```python
from build123d import *

# Parameters (mm, degrees)
SKETCH1_W                   = 89
SKETCH1_H                   = 83
SKETCH1_R                   = 1.3
MAIN_BODY_DEPTH             = 14
SKETCH2_W                   = 73.025
SKETCH2_H                   = 83
SKETCH2_R                   = 4
SCREW_RISER_DEPTH           = 2
SKETCH4_W                   = 7.9875
SKETCH4_H                   = 83
TOPPER_SUPPORT_DEPTH        = 20
MOUNT_START                 = -44.5
MOUNT_NUTS_DEPTH            = 41.275
F_9_32_MOUNT_HOLES_REACH    = 9.988
SKETCH5_R                   = 3.3734375
SKETCH8_W                   = 19.0125
SKETCH8_H                   = 43
MIDDLE_CUT_DEPTH            = 14
SKETCH9_R                   = 3.3734375
MOUNT_NUTS_P2_DEPTH         = 4.7625
SKETCH9_3_R                 = 3.3734375
F_9_32_MOUNT_HOLES_P2_DEPTH = 7.9875


with BuildPart() as part:
    # Sketch1 → Main Body (new body)
    with BuildSketch(Plane(origin=(0, 0, 0), x_dir=(1, 0, 0), z_dir=(0, 1, 0))):
        with Locations((0, 41.5)):
            Rectangle(SKETCH1_W, SKETCH1_H)
        with Locations((-30, 14.25)):
            Circle(SKETCH1_R, mode=Mode.SUBTRACT)
        with Locations((30, 14.25)):
            Circle(SKETCH1_R, mode=Mode.SUBTRACT)
        with BuildLine():
            Line((-7.5, 12.5), (-7.5, 70.5))
            ThreePointArc((-7.5, 70.5), (0, 78), (7.5, 70.5))
            Line((7.5, 70.5), (7.5, 12.5))
            ThreePointArc((7.5, 12.5), (0, 5), (-7.5, 12.5))
        make_face(mode=Mode.SUBTRACT)
        with Locations((-30, 68.75)):
            Circle(SKETCH1_R, mode=Mode.SUBTRACT)
        with Locations((30, 68.75)):
            Circle(SKETCH1_R, mode=Mode.SUBTRACT)
    extrude(amount=MAIN_BODY_DEPTH)

    # Sketch2 → Screw Riser (cut)
    with BuildSketch(Plane(origin=(0, 14, 0), x_dir=(1, 0, 0), z_dir=(0, 1, 0))):
        with Locations((0, 41.5)):
            Rectangle(SKETCH2_W, SKETCH2_H)
        with Locations((-30, 14.25)):
            Circle(SKETCH2_R, mode=Mode.SUBTRACT)
        with Locations((30, 14.25)):
            Circle(SKETCH2_R, mode=Mode.SUBTRACT)
        with Locations((-30, 68.75)):
            Circle(SKETCH2_R, mode=Mode.SUBTRACT)
        with Locations((30, 68.75)):
            Circle(SKETCH2_R, mode=Mode.SUBTRACT)
    extrude(amount=-SCREW_RISER_DEPTH, mode=Mode.SUBTRACT)

    # Sketch4 → Topper Support (add)
    with BuildSketch(Plane(origin=(0, 14, 0), x_dir=(1, 0, 0), z_dir=(0, 1, 0))):
        with Locations((-40.50625, 41.5)):
            Rectangle(SKETCH4_W, SKETCH4_H)
        with Locations((40.50625, 41.5)):
            Rectangle(SKETCH4_W, SKETCH4_H)
    extrude(amount=TOPPER_SUPPORT_DEPTH)

    # Sketch6 → Mount Nuts (cut)
    with BuildSketch(Plane.ZY.offset(44.5).offset(MOUNT_START)):
        Polygon((-52.96962719, 22.65546875), (-56.234813595, 28.3109375), (-62.765186405, 28.3109375), (-66.03037281, 22.65546875), (-62.765186405, 17), (-56.234813595, 17), align=None)
        Polygon((-16.96962719, 22.65546875), (-20.234813595, 28.3109375), (-26.765186405, 28.3109375), (-30.03037281, 22.65546875), (-26.765186405, 17), (-20.234813595, 17), align=None)
    extrude(amount=MOUNT_NUTS_DEPTH, mode=Mode.SUBTRACT)

    # Sketch5 → 9/32 Mount Holes (cut, up to next)
    with BuildSketch(Plane.ZY.offset(36.5125), mode=Mode.PRIVATE) as f_9_32_mount_holes_sk1:
        with Locations((-59.5, 22.65546875)):
            Circle(SKETCH5_R)
    f_9_32_mount_holes_tool1 = extrude(f_9_32_mount_holes_sk1.sketch, amount=F_9_32_MOUNT_HOLES_REACH, mode=Mode.PRIVATE) & part.part
    add(f_9_32_mount_holes_tool1.solids().sort_by_distance((-36.5125, 22.655469, -59.5))[0], mode=Mode.SUBTRACT)
    # Sketch5 → 9/32 Mount Holes (cut, up to next)
    with BuildSketch(Plane.ZY.offset(36.5125), mode=Mode.PRIVATE) as f_9_32_mount_holes_sk2:
        with Locations((-23.5, 22.65546875)):
            Circle(SKETCH5_R)
    f_9_32_mount_holes_tool2 = extrude(f_9_32_mount_holes_sk2.sketch, amount=F_9_32_MOUNT_HOLES_REACH, mode=Mode.PRIVATE) & part.part
    add(f_9_32_mount_holes_tool2.solids().sort_by_distance((-36.5125, 22.655469, -23.5))[0], mode=Mode.SUBTRACT)

    # Sketch8 → Middle Cut (cut)
    with BuildSketch(Plane(origin=(0, 14, 0), x_dir=(1, 0, 0), z_dir=(0, 1, 0))):
        with Locations((-27.00625, 41.5)):
            Rectangle(SKETCH8_W, SKETCH8_H)
        with Locations((27.00625, 41.5)):
            Rectangle(SKETCH8_W, SKETCH8_H)
    extrude(amount=-MIDDLE_CUT_DEPTH, mode=Mode.SUBTRACT)

    # Sketch9 → Mount Nuts p2 (cut)
    with BuildSketch(Plane.ZY.offset(-36.5125)):
        Polygon((-56.234813595, 17), (-62.765186405, 17), (-66.03037281, 22.65546875), (-62.765186405, 28.3109375), (-56.234813595, 28.3109375), (-52.96962719, 22.65546875), align=None)
        with Locations((-59.5, 22.65546875)):
            Circle(SKETCH9_R, mode=Mode.SUBTRACT)
        with Locations((-59.5, 22.65546875)):
            Circle(SKETCH9_R)
        Polygon((-20.234813595, 17), (-26.765186405, 17), (-30.03037281, 22.65546875), (-26.765186405, 28.3109375), (-20.234813595, 28.3109375), (-16.96962719, 22.65546875), align=None)
        with Locations((-23.5, 22.65546875)):
            Circle(SKETCH9_R, mode=Mode.SUBTRACT)
        with Locations((-23.5, 22.65546875)):
            Circle(SKETCH9_R)
    extrude(amount=-MOUNT_NUTS_P2_DEPTH, mode=Mode.SUBTRACT)

    # Sketch9<3> → 9/32 Mount Holes p2 (cut)
    with BuildSketch(Plane.ZY.offset(-36.5125)):
        with Locations((-59.5, 22.65546875)):
            Circle(SKETCH9_3_R)
        with Locations((-23.5, 22.65546875)):
            Circle(SKETCH9_3_R)
    extrude(amount=-F_9_32_MOUNT_HOLES_P2_DEPTH, mode=Mode.SUBTRACT)


solid = part.part
```
Model file for the job. Use its own axes, mm. A direction names the side the tool comes from. Coordinates: 2 decimals unless noted, no trailing zeros. Write each loop counter-clockwise with the first axis right and the second up, starting at its lowest first coordinate (ties: lowest second). Pieces come first, ordered by that corner, then holes. Notation, with made-up numbers: (-3, 49) - (1, 49) arc R12 ccw to (1, 55) - close; hole circle Ø4 at (79.5, 55.25). An arc over 180 degrees is marked (long way). One line per item, written item: value. Start each with the question number.
1. Mould opens along X. For faces 4 (the flat face through (36.512, 17, -41)), 5 (the flat face through (44.5, 17, -41)), 6 (the flat face through (17.5, 6, -41)), 7 (the flat face through (40, 34, -42)) say: released by +X, released by -X, zero draft, split by the parting line, or undercut.
2. Tool access for faces 1 (the flat face through (-27, 6, -63)), 2 (the flat face through (-41.275, 20, -57)), 3 (the cylindrical face through (42.865, 21.363, -56.384)): list every direction of +Z, -Z, +X, -X, +Y, -Y with a clear straight run to the whole face (end or side of a thin tool).
3. Flat gauge pins, fed straight in: pin 1 (5.5 mm diameter, centred on y = 22.66, z = -59.5, fed in from -X); pin 2 (10 mm diameter, centred on x = 8.5, z = -21.5, fed in from +Y); pin 3 (9 mm diameter, centred on x = 29, z = -13, fed in from +Y). Where does each tip first touch, or does it go through?
4. Slice it at A-A (x = 30). Write the cut outline in (y, z), plus the area to 3 significant figures.
5. Slice it at B-B (z = -23.5). Count the separate pieces of the cut face and the enclosed holes in it, plus the area to 3 significant figures.
6. Probe line 1 (X direction, y = 9.5, z = -14.25); line 2 (X direction, y = 3.5, z = -22); line 3 (Z direction, x = -30, y = 4). List the from-to ranges inside material, lowest first. Write a range as from..to.
7. Slice it at C-C (x = 0). Write the cut outline in (y, z).
8. Slice it at D-D (y = 3). Write the cut outline in (x, z).
Answers below:
1. face 4: undercut
1. face 5: released by +X
1. face 6: undercut
1. face 7: zero draft
2. face 1: +Y, -Y
2. face 2: none
2. face 3: +X, -X
3. pin 1: passes through
3. pin 2: stops at y = 12
3. pin 3: stops at y = 14
4. outline: (0, -83) - (12, -83) - (12, -72.75) - (14, -72.75) - (14, -70.05) - (0, -70.05) - close; (0, -67.45) - (14, -67.45) - (14, -64.75) - (12, -64.75) - (12, -63) - (0, -63) - close; (0, -20) - (12, -20) - (12, -18.25) - (14, -18.25) - (14, -15.55) - (0, -15.55) - close; (0, -12.95) - (14, -12.95) - (14, -10.25) - (12, -10.25) - (12, 0) - (0, 0) - close
4. area: 439 mm^2
5. separate pieces: 6
5. enclosed holes: 0
5. area: 632 mm^2
6. line 1: x = -44.5..-31.3, -28.7..-7.5, 7.5..28.7, 31.3..44.5
6. line 2: x = -44.5..-36.51, -17.5..-7.5, 7.5..17.5, 36.51..44.5
6. line 3: z = -83..-70.05, -67.45..-63, -20..-15.55, -12.95..0
7. outline: (0, -83) - (12, -83) - (12, -78) - (0, -78) - close; (0, -5) - (12, -5) - (12, 0) - (0, 0) - close
8. outline: (-44.5, -83) - (44.5, -83) - (44.5, 0) - (-44.5, 0) - close; hole (-36.51, -63) - (-17.5, -63) - (-17.5, -20) - (-36.51, -20) - close; hole circle Ø2.6 at (-30, -68.75); hole circle Ø2.6 at (-30, -14.25); hole (-7.5, -70.5) arc R7.5 ccw to (7.5, -70.5) - (7.5, -12.5) arc R7.5 ccw to (-7.5, -12.5) - close; hole (17.5, -63) - (36.51, -63) - (36.51, -20) - (17.5, -20) - close; hole circle Ø2.6 at (30, -68.75); hole circle Ø2.6 at (30, -14.25)
